Geometry check sheet. Reference: the model listing, model coordinates, mm. A direction names the side the tool comes from. Coordinates: 2 decimals unless noted, no trailing zeros. Order: outer loops, then holes, each group sorted by start corner. A loop starts at its lowest first (then second) coordinate and runs counter-clockwise, first axis right, second up. Notation, with made-up numbers: (61, 79) - (118, 79) arc R23 ccw to (118, 88) - close; hole circle Ø4 at (71, -12.75). An arc over 180 degrees is marked (long way). Put each result on its own line as item: value.
from build123d import *

# Parameters (mm, degrees)
BOSS_EXTRU_1_DEPTH         = 40
ESQUISSE1_R                = 1
ENL_V_MAT_EXTRU_1_DEPTH    = 6.695841166
R_P_TITION_LIN_AIRE2_COUNT = 2
R_P_TITION_LIN_AIRE2_PITCH = 20


with BuildPart() as part:
    # ProfileRainureEsquisse → Boss.-Extru.1 (new body)
    with BuildSketch(Plane.XY):
        Polygon((0, 0), (0, 5), (4, 8), (4, 5), (5.695841166, 5), (5.695841166, 0), (4, 0), (4, -3), align=None)
    extrude(amount=BOSS_EXTRU_1_DEPTH)

    # Esquisse1 → Enlèv. mat.-Extru.1 (cut, through all)
    with BuildSketch(Plane(origin=(5.695841166, 0, 0), x_dir=(0, 0, -1), z_dir=(1, 0, 0))):
        with Locations((-30, 2.5)):
            Circle(ESQUISSE1_R)
    enl_v_mat_extru_1 = extrude(amount=-ENL_V_MAT_EXTRU_1_DEPTH, mode=Mode.SUBTRACT)

    # Répétition linéaire2: Enlèv. mat.-Extru.1 ×2
    with Locations(*[(0, 0, -i * R_P_TITION_LIN_AIRE2_PITCH) for i in range(1, R_P_TITION_LIN_AIRE2_COUNT)]):
        add(enl_v_mat_extru_1, mode=Mode.SUBTRACT)


solid = part.part
Q1. Draft check along Y on faces 1 (the flat face through (5, 0, 20)), 2 (the cylindrical face through (2.9, 2.5, 11)), 3 (the flat face through (0, 2, 20)). Enter one of: pulls with the +Y half, pulls with the -Y half, needs draft (parallel to the pull), parting line crosses it, or undercut.
Answer block:
face 1: pulls with the -Y half
face 2: undercut
face 3: needs draft
Q2. Section check D-D on z = 20.5. Record the boundary of the cut face in (x, y).
Answer block:
outline: (0, 0) - (4, -3) - (4, 0) - (5.7, 0) - (5.7, 5) - (4, 5) - (4, 8) - (0, 5) - close
Q3. Thickness scan on L1, parallel to Y at x = 4.45, z = 30; L2, parallel to Y at x = 1.7, z = 30 (3 decimals); L3, parallel to Z at x = 4.9, y = 3. Record the ranges inside material, lowest first. Write a range as [from, to].
Answer block:
L1: y = [0, 1.5], [3.5, 5]
L2: y = [-1.275, 1.5], [3.5, 6.275]
L3: z = [0, 9.13], [10.87, 29.13], [30.87, 40]
Q4. Section check A-A on z = 30. Record the boundary of the cut face in (x, y), then the cut area to 3 significant figures.
Answer block:
outline: (0, 0) - (4, -3) - (4, 0) - (5.7, 0) - (5.7, 1.5) - (0, 1.5) - close; (0, 3.5) - (5.7, 3.5) - (5.7, 5) - (4, 5) - (4, 8) - (0, 5) - close
area: 29.1 mm^2
Q5. Access from +Z, -Z, +X, -X, +Y, -Y to the whole of each face (thin tool, end or side, straight path). Record for faces 4 (the flat face through (5, 5, 20)), 5 (the flat face through (2, -1.5, 19.7)), 6 (the flat face through (4, -1, 20)).
Answer block:
face 4: +Z, -Z, +X, +Y
face 5: +Z, -Z, -X, -Y
face 6: +Z, -Z, +X, -Y
Q6. Depth check by flat-ended pin: pin 1 Ø1.8 at (y, z) = (2.5, 30) entering from +X; pin 2 Ø0.5 at (x, z) = (4.5, 14) entering from -Y; pin 3 Ø2.5 at (y, z) = (-1.5, 26.5) entering from +X; pin 4 Ø0.8 at (x, z) = (4.5, 11.5) entering from +Y. Enter the tip coordinate at first touch or a pass-through.
Answer block:
pin 1: passes through
pin 2: stops at y = 0
pin 3: stops at x = 4
pin 4: stops at y = 5
Q7. Section check C-C on y = 2. Record the boundary of the cut face in (x, z), then the cut area to 3 significant figures.
Answer block:
outline: (0, 0) - (5.7, 0) - (5.7, 9.13) - (0, 9.13) - close; (0, 10.87) - (5.7, 10.87) - (5.7, 29.13) - (0, 29.13) - close; (0, 30.87) - (5.7, 30.87) - (5.7, 40) - (0, 40) - close
area: 208 mm^2
Q8. Section check B-B on x = 5. Record the boundary of the cut face in (y, z).
Answer block:
outline: (0, 0) - (5, 0) - (5, 40) - (0, 40) - close; hole circle Ø2 at (2.5, 10); hole circle Ø2 at (2.5, 30)
